Read the model definition and answer for the solid it produces. Units are mm, in the model's axes. A direction names the side the tool comes from. Coordinates: 2 decimals unless noted, no trailing zeros. Loops run counter-clockwise (first coordinate to the right, second up) from the corner with the lowest first, then second, coordinate; pieces in that order, holes last. Notation, with made-up numbers: M 7.25,9 L 48.25,9 A16 cw 48.25,34 Z; hole C 5,43 d4. An arc over 180 degrees is marked long. One line per item, written item: value. Start each with the question number.
1. The part is cut by section A-A (y = 3.5). Write down the section's boundary in (x, z), then the cut area to 3 significant figures.
2. Flat-ended cylindrical pins translate along their axes: pin 1 (0.5 mm diameter, centred on x = -4, z = 3.5, fed in from +Y); pin 2 (0.5 mm diameter, centred on x = 4.5, y = 7.5, fed in from -Z); pin 3 (12 mm diameter, centred on y = -9, z = 26.5, fed in from -X); pin 4 (1.9 mm diameter, centred on x = 1.5, z = 20.5, fed in from +Y). Find the tip coordinate at first contact, or state that the pin passes through.
3. The part is cut by section C-C (z = 16.5). Write down the section's boundary in (x, y) (3 decimals).
4. The part is cut by section B-B (z = 31.75). Write down the section's boundary in (x, y) (3 decimals), then the cut area to 3 significant figures.
5. For faces 5 (the face through (-4, 9, 4.826)), 6 (the face through (7, 8, 3.048)), 7 (the face through (4, -4, 7.366)), 8 (the face through (6, 17.78, 6)), determine the directions among +Z, -Z, +X, -X, +Y, -Y from which every point of the face is accessible in a straight line to the end or side of a thin tool.
6. Consider probe 1 along Z at (x, y) = (6.5, 5.5); probe 2 along Z at (x, y) = (0.75, -18.5); probe 3 along X at (y, z) = (-18, 32). Determine where each line is inside the solid, lowest interval first.
7. The part is cut by section D-D (z = -29.5). Write down the section's boundary in (x, y) (3 decimals), then the cut area to 3 significant figures.
8. Determine the mould class of faces 1 (the face through (-3.556, 5, 6)), 2 (the face through (-6.4, -3.29, -0.04)), 3 (the face through (0, -19, 38.1)), 4 (the face through (4, -4, -7.366)) for opening direction Z: +Z half, -Z half, draft (parallel to the pull), parting line (faces both ways), or undercut.
```python
from build123d import *

# Parameters (mm, degrees)
BOSS_EXTRUDE1_DEPTH            = 17.78
BOSS_EXTRUDE1_2_DEPTH          = 17.78
BOSS_EXTRUDE1_3_DEPTH          = 17.78
BOSS_EXTRUDE1_4_DEPTH          = 17.78
SKETCH2_W                      = 15.748
SKETCH2_H                      = 14.732
BOSS_EXTRUDE2_DEPTH            = 17.78
SKETCH3_W                      = 15.748
SKETCH3_H                      = 76.2
SKETCH3_R                      = 3.429
BOSS_EXTRUDE3_DEPTH            = 3.175
CUT_EXTRUDE3_DEPTH             = 0.635
CUT_EXTRUDE4_REACH             = 46.19
CUT_EXTRUDE4_DIRECTION_2_REACH = 46.19
CUT_EXTRUDE5_REACH             = 46.19
CUT_EXTRUDE5_DIRECTION_2_REACH = 46.19


with BuildPart() as part:
    # Sketch1 → Boss-Extrude1 (new body)
    with BuildSketch(Plane(origin=(0, 0, 0), x_dir=(1, 0, 0), z_dir=(0, 1, 0))):
        Polygon((-5.334, 4.826), (-5.334, 3.048), (-7.874, 3.048), (-7.874, 7.366), (-3.556, 7.366), (-3.556, 4.826), align=None)
    extrude(amount=BOSS_EXTRUDE1_DEPTH)



with BuildPart() as body_2:
    # Sketch1 → Boss-Extrude1 2 (new body)
    with BuildSketch(Plane(origin=(0, 0, 0), x_dir=(1, 0, 0), z_dir=(0, 1, 0))):
        Polygon((7.874, 3.048), (7.874, 7.366), (3.556, 7.366), (3.556, 4.826), (5.334, 4.826), (5.334, 3.048), align=None)
    extrude(amount=BOSS_EXTRUDE1_2_DEPTH)


with BuildPart() as body_3:
    # Sketch1 → Boss-Extrude1 3 (new body)
    with BuildSketch(Plane(origin=(0, 0, 0), x_dir=(1, 0, 0), z_dir=(0, 1, 0))):
        Polygon((5.334, -3.048), (7.874, -3.048), (7.874, -7.366), (3.556, -7.366), (3.556, -4.826), (5.334, -4.826), align=None)
    extrude(amount=BOSS_EXTRUDE1_3_DEPTH)


with BuildPart() as body_4:
    # Sketch1 → Boss-Extrude1 4 (new body)
    with BuildSketch(Plane(origin=(0, 0, 0), x_dir=(1, 0, 0), z_dir=(0, 1, 0))):
        Polygon((-5.334, -3.048), (-7.874, -3.048), (-7.874, -7.366), (-3.556, -7.366), (-3.556, -4.826), (-5.334, -4.826), align=None)
    extrude(amount=BOSS_EXTRUDE1_4_DEPTH)


with BuildPart() as part_1:
    add(part.part)

    add(body_2.part)  # Boss-Extrude2 merges body 2

    add(body_3.part)  # Boss-Extrude2 merges body 3

    add(body_4.part)  # Boss-Extrude2 merges body 4
    # Sketch2 → Boss-Extrude2 (add)
    with BuildSketch(Plane(origin=(0, 0, 0), x_dir=(-1, 0, 0), z_dir=(0, -1, 0))):
        Rectangle(SKETCH2_W, SKETCH2_H)
    extrude(amount=BOSS_EXTRUDE2_DEPTH)

    # Sketch3 → Boss-Extrude3 (add)
    with BuildSketch(Plane(origin=(0, -17.78, 0), x_dir=(-1, 0, 0), z_dir=(0, -1, 0))):
        Rectangle(SKETCH3_W, SKETCH3_H)
        with Locations(Location((0, 31.75, 0), (0, 0, 90))):
            Circle(SKETCH3_R, mode=Mode.SUBTRACT)
        with Locations(Location((0, -31.75, 0), (0, 0, 270))):
            Circle(SKETCH3_R, mode=Mode.SUBTRACT)
    extrude(amount=BOSS_EXTRUDE3_DEPTH)

    # Sketch5 → Cut-Extrude3 (cut)
    with BuildSketch(Plane(origin=(0, -17.78, 0), x_dir=(1, 0, 0), z_dir=(0, 1, 0))):
        Polygon((-4.402938034, -19.56265828), (-3.33951656, -19.56265828), (-2.238782051, -22.073125862), (-1.138047543, -19.56265828), (-0.074626068, -19.56265828), (-1.937945713, -23.816344178), (-2.539618389, -23.816344178), align=None)
        with BuildLine():
            Line((1.342103198, -17.995510844), (3.992494658, -17.995510844))
            Line((3.992494658, -17.995510844), (3.992494658, -18.965649733))
            Line((3.992494658, -18.965649733), (2.169986144, -18.965649733))
            Line((2.169986144, -18.965649733), (1.942609842, -20.066384242))
            add(Edge.make_bspline(
                [(1.942609842, -20.066384242), (1.973593118, -20.057755008), (2.034698504, -20.040736387), (2.126753844, -20.023668863), (2.215968297, -20.012606236), (2.274510277, -20.011130629), (2.302913829, -20.01041469)],
                knots=[0, 0, 0, 0, 1.05461699, 2.079921384, 3.068411212, 4, 4, 4, 4], degree=3))
            add(Edge.make_bspline(
                [(2.302913829, -20.01041469), (2.364808143, -20.011832963), (2.486815471, -20.01462869), (2.66529671, -20.04116926), (2.83620304, -20.082969854), (2.999011469, -20.142586126), (3.153562954, -20.220178243), (3.300044843, -20.314042954), (3.438636917, -20.42434512), (3.566877199, -20.551153798), (3.684709726, -20.690392598), (3.787158388, -20.840994093), (3.874655939, -21.000810853), (3.944248465, -21.170836295), (3.99917682, -21.350002545), (4.038869276, -21.538424417), (4.062341408, -21.736325221), (4.065506481, -21.87133879), (4.067120726, -21.940198177)],
                knots=[0, 0, 0, 0, 1.01440847, 1.999622559, 2.951875003, 3.895578053, 4.836219714, 5.782137149, 6.743708247, 7.735272588, 8.734977101, 9.730283169, 10.717124674, 11.717316708, 12.737475749, 13.78628267, 14.87096371, 16, 16, 16, 16], degree=3))
            add(Edge.make_bspline(
                [(4.067120726, -21.940198177), (4.065148093, -22.009839278), (4.061255511, -22.147261527), (4.035859977, -22.349320843), (3.991036403, -22.542848052), (3.92946674, -22.728361222), (3.848352651, -22.904496875), (3.750801857, -23.073079646), (3.635165037, -23.232858198), (3.502576985, -23.382194608), (3.358436381, -23.518690953), (3.204960663, -23.63876705), (3.043228044, -23.739810112), (2.873234622, -23.821469989), (2.695955704, -23.88607783), (2.511337482, -23.933109254), (2.318482737, -23.960079163), (2.187559423, -23.963737055), (2.121012787, -23.965596314)],
                knots=[0, 0, 0, 0, 1.06808661, 2.107647099, 3.116961351, 4.110378221, 5.100014249, 6.085620622, 7.093190682, 8.119403071, 9.144090782, 10.133780668, 11.103064255, 12.062861538, 13.020824475, 13.992378307, 14.979551724, 16, 16, 16, 16], degree=3))
            add(Edge.make_bspline(
                [(2.121012787, -23.965596314), (2.061502111, -23.964075324), (1.944134605, -23.961075614), (1.77125742, -23.942637813), (1.604584616, -23.910039607), (1.445001044, -23.862861563), (1.290827618, -23.804796161), (1.143846625, -23.732174402), (1.003250382, -23.646379103), (0.869438127, -23.54897603), (0.744584119, -23.439255246), (0.630630611, -23.319146944), (0.526887714, -23.19016503), (0.435575361, -23.050718259), (0.356979792, -22.901012655), (0.287279637, -22.742812535), (0.230229362, -22.574465784), (0.201277991, -22.457758463), (0.186565171, -22.398448878)],
                knots=[0, 0, 0, 0, 1.054957082, 2.080596141, 3.077793124, 4.061112343, 5.027190972, 5.994718051, 6.962465889, 7.943658696, 8.924948258, 9.904494768, 10.875059, 11.855380583, 12.854004648, 13.869083016, 14.917087635, 16, 16, 16, 16], degree=3))
            Line((0.186565171, -22.398448878), (1.380582265, -22.398448878))
            add(Edge.make_bspline(
                [(1.380582265, -22.398448878), (1.402408926, -22.439548005), (1.444826552, -22.519419468), (1.525514253, -22.625460837), (1.615839012, -22.71588836), (1.71498605, -22.791585534), (1.823597778, -22.848296569), (1.937248474, -22.891303595), (2.057365883, -22.916155762), (2.139171142, -22.919262529), (2.180480435, -22.920831357)],
                knots=[0, 0, 0, 0, 1.104910296, 2.147267069, 3.153527244, 4.136738762, 5.099945312, 6.05603338, 7.018353, 8, 8, 8, 8], degree=3))
            add(Edge.make_bspline(
                [(2.180480435, -22.920831357), (2.209272459, -22.919748068), (2.265921249, -22.917616678), (2.349384285, -22.906341091), (2.429053419, -22.884985384), (2.505520973, -22.855412696), (2.578992357, -22.818532212), (2.648414335, -22.771973005), (2.714994724, -22.718381632), (2.777719899, -22.656885349), (2.834530829, -22.588331299), (2.884347799, -22.514665298), (2.928891041, -22.437524221), (2.961884902, -22.353852317), (2.988904083, -22.266148059), (3.008802101, -22.173749865), (3.020693411, -22.076549824), (3.021794228, -22.01019408), (3.022355769, -21.976345179)],
                knots=[0, 0, 0, 0, 0.978869489, 1.925942215, 2.855067702, 3.774946051, 4.70828698, 5.642468714, 6.60995405, 7.609372294, 8.622401667, 9.629904756, 10.629323, 11.642352373, 12.678539694, 13.745912462, 14.850161547, 16, 16, 16, 16], degree=3))
            add(Edge.make_bspline(
                [(3.022355769, -21.976345179), (3.021704036, -21.943281988), (3.020435422, -21.878923684), (3.009941194, -21.784422641), (2.99116722, -21.694758253), (2.965587521, -21.609243759), (2.932842452, -21.528398443), (2.892825789, -21.451741076), (2.845366576, -21.379659132), (2.790210015, -21.31362013), (2.731391627, -21.253047278), (2.668201777, -21.200070745), (2.601209774, -21.156103901), (2.532497311, -21.117719567), (2.459321633, -21.089784285), (2.383328169, -21.070546287), (2.304596835, -21.056430218), (2.250895901, -21.055600847), (2.223623631, -21.055179648)],
                knots=[0, 0, 0, 0, 1.166249705, 2.270133367, 3.348514167, 4.393962215, 5.415026464, 6.420877785, 7.440098956, 8.453121383, 9.451844239, 10.415694839, 11.355045125, 12.27538808, 13.187007209, 14.108269027, 15.039275622, 16, 16, 16, 16], degree=3))
            add(Edge.make_bspline(
                [(2.223623631, -21.055179648), (2.193999608, -21.056303715), (2.13462671, -21.058556587), (2.046413445, -21.076887601), (1.959263786, -21.106554059), (1.872693092, -21.14748364), (1.787560727, -21.201047546), (1.701620007, -21.263871867), (1.617747551, -21.340521386), (1.56441911, -21.397610121), (1.536830596, -21.427143957)],
                knots=[0, 0, 0, 0, 0.88288272, 1.769486374, 2.674910571, 3.623812639, 4.617874466, 5.670434592, 6.794841017, 8, 8, 8, 8], degree=3))
            Line((1.536830596, -21.427143957), (0.657642228, -21.225420366))
            Line((0.657642228, -21.225420366), (1.342103198, -17.995510844))
        make_face()
    extrude(amount=-CUT_EXTRUDE3_DEPTH, mode=Mode.SUBTRACT)

    # Cut-Extrude4: up to this face of the body (flat: up to its plane)
    cut_extrude4_end = Plane(part_1.part.faces().sort_by_distance((-3.556, 8.89, 6.096))[0])
    # Sketch6 → Cut-Extrude4 (cut, up to the picked face)
    with BuildSketch(Plane(origin=(0, 0, 0), x_dir=(0, 0, -1), z_dir=(1, 0, 0)), mode=Mode.PRIVATE) as cut_extrude4_sk1:
        with BuildLine():
            Line((-7.366, -7.366), (-7.366, 2.54))
            Line((-7.366, 2.54), (7.366, 2.54))
            Line((7.366, 2.54), (7.366, -7.366))
            ThreePointArc((7.366, -7.366), (0, 0), (-7.366, -7.366))
        make_face()
    cut_extrude4_tool1 = split(extrude(cut_extrude4_sk1.sketch, amount=-CUT_EXTRUDE4_REACH, mode=Mode.PRIVATE), bisect_by=cut_extrude4_end, keep=Keep.BOTH, mode=Mode.PRIVATE)
    add(cut_extrude4_tool1.solids().sort_by(Axis((0, 0.151656, 0), (-1, 0, 0)))[0], mode=Mode.SUBTRACT)

    # Cut-Extrude4 direction 2: up to this face of the body (flat: up to its plane)
    cut_extrude4_direction_2_end = Plane(part_1.part.faces().sort_by_distance((3.556, 8.89, 6.096))[0])
    # Sketch6 → Cut-Extrude4 direction 2 (cut, up to the picked face)
    with BuildSketch(Plane(origin=(0, 0, 0), x_dir=(0, 0, -1), z_dir=(1, 0, 0)), mode=Mode.PRIVATE) as cut_extrude4_direction_2_sk1:
        with BuildLine():
            Line((-7.366, -7.366), (-7.366, 2.54))
            Line((-7.366, 2.54), (7.366, 2.54))
            Line((7.366, 2.54), (7.366, -7.366))
            ThreePointArc((7.366, -7.366), (0, 0), (-7.366, -7.366))
        make_face()
    cut_extrude4_direction_2_tool1 = split(extrude(cut_extrude4_direction_2_sk1.sketch, amount=CUT_EXTRUDE4_DIRECTION_2_REACH, mode=Mode.PRIVATE), bisect_by=cut_extrude4_direction_2_end, keep=Keep.BOTH, mode=Mode.PRIVATE)
    add(cut_extrude4_direction_2_tool1.solids().sort_by(Axis((0, 0.151656, 0), (1, 0, 0)))[0], mode=Mode.SUBTRACT)

    # Cut-Extrude5: up to this face of the body (flat: up to its plane)
    cut_extrude5_end = Plane(part_1.part.faces().sort_by_distance((-6.604, 8.89, -3.048))[0])
    # Sketch7 → Cut-Extrude5 (cut, up to the picked face)
    with BuildSketch(Plane.XY, mode=Mode.PRIVATE) as cut_extrude5_sk1:
        with BuildLine():
            Line((-7.874, -7.874), (-7.874, 4.538671937))
            Line((-7.874, 4.538671937), (7.874, 4.538671937))
            Line((7.874, 4.538671937), (7.874, -7.874))
            ThreePointArc((7.874, -7.874), (0, 0), (-7.874, -7.874))
        make_face()
    cut_extrude5_tool1 = split(extrude(cut_extrude5_sk1.sketch, amount=-CUT_EXTRUDE5_REACH, mode=Mode.PRIVATE), bisect_by=cut_extrude5_end, keep=Keep.BOTH, mode=Mode.PRIVATE)
    add(cut_extrude5_tool1.solids().sort_by(Axis((0, 1.176505, 0), (0, 0, -1)))[0], mode=Mode.SUBTRACT)

    # Cut-Extrude5 direction 2: up to this face of the body (flat: up to its plane)
    cut_extrude5_direction_2_end = Plane(part_1.part.faces().sort_by_distance((-6.604, 8.89, 3.048))[0])
    # Sketch7 → Cut-Extrude5 direction 2 (cut, up to the picked face)
    with BuildSketch(Plane.XY, mode=Mode.PRIVATE) as cut_extrude5_direction_2_sk1:
        with BuildLine():
            Line((-7.874, -7.874), (-7.874, 4.538671937))
            Line((-7.874, 4.538671937), (7.874, 4.538671937))
            Line((7.874, 4.538671937), (7.874, -7.874))
            ThreePointArc((7.874, -7.874), (0, 0), (-7.874, -7.874))
        make_face()
    cut_extrude5_direction_2_tool1 = split(extrude(cut_extrude5_direction_2_sk1.sketch, amount=CUT_EXTRUDE5_DIRECTION_2_REACH, mode=Mode.PRIVATE), bisect_by=cut_extrude5_direction_2_end, keep=Keep.BOTH, mode=Mode.PRIVATE)
    add(cut_extrude5_direction_2_tool1.solids().sort_by(Axis((0, 1.176505, 0), (0, 0, 1)))[0], mode=Mode.SUBTRACT)


solid = part_1.part
```
Answer block:
1. outline: M -7.87,-7.37 L -3.56,-7.37 L -3.56,-4.83 L -5.33,-4.83 L -5.33,-3.05 L -7.87,-3.05 Z; M -7.87,3.05 L -5.33,3.05 L -5.33,4.83 L -3.56,4.83 L -3.56,7.37 L -7.87,7.37 Z; M 3.56,-7.37 L 7.87,-7.37 L 7.87,-3.05 L 5.33,-3.05 L 5.33,-4.83 L 3.56,-4.83 Z; M 3.56,4.83 L 5.33,4.83 L 5.33,3.05 L 7.87,3.05 L 7.87,7.37 L 3.56,7.37 Z
1. area: 61.9 mm2
2. pin 1: stops at y = 0
2. pin 2: stops at z = -7.37
2. pin 3: passes through
2. pin 4: stops at y = -17.78
3. outline: M -7.874,-20.955 L 7.874,-20.955 L 7.874,-17.78 L -7.874,-17.78 Z
4. outline: M -7.874,-20.955 L -3.429,-20.955 L -3.429,-17.78 L -7.874,-17.78 Z; M 3.429,-20.955 L 7.874,-20.955 L 7.874,-17.78 L 3.429,-17.78 Z
4. area: 28.2 mm2
5. face 5: +Y
5. face 6: +X, +Y
5. face 7: +Z, +X, -X, +Y
5. face 8: +Z, -Z, +X, -X, +Y
6. probe 1: z = -7.37 to -3.05, 3.05 to 7.37
6. probe 2: z = -38.1 to -35.1, -28.4 to 28.4, 35.1 to 38.1
6. probe 3: x = -7.87 to -3.42, 3.42 to 7.87
7. outline: M -7.874,-20.955 L -2.588,-20.955 L -2.588,-17.78 L -7.874,-17.78 Z; M 2.588,-20.955 L 7.874,-20.955 L 7.874,-17.78 L 2.588,-17.78 Z
7. area: 33.6 mm2
8. face 1: draft
8. face 2: undercut
8. face 3: +Z half
8. face 4: -Z half
